The listing builds one solid part. Answer for the finished solid, in the listing's coordinates (mm). Round coordinates to 2 decimals unless told otherwise and drop trailing zeros. Write each loop counter-clockwise with the first axis right and the second up, starting at its lowest first coordinate (ties: lowest second). Pieces come first, ordered by that corner, then holes. Notation, with made-up numbers: M 68,-23.75 L 116,-23.75 A19 cw 116,-0.75 Z; hole C -16,46.25 d7. An arc over 180 degrees is marked long. One line per item, written item: value. Start each with the question number.
(1) Section D-D (z = -26.5) is taken. Determine the outline of the cut face in (x, y), plus the area to 3 significant figures.
(2) Section C-C (y = 14.25) is taken. Determine the outline of the cut face in (x, z).
(3) Section B-B (z = 0) is taken. Determine the outline of the cut face in (x, y).
(4) Consider probe 1 along Z at (x, y) = (0, 10.5); probe 2 along Z at (x, y) = (26, 16.25); probe 3 along X at (y, z) = (3.5, -16.5). Determine where each line is inside the solid, lowest interval first.
(5) Given P1, Ø3, axis at x = 0, z = -8, coming from the -Y side; P2, Ø8, axis at x = -32, y = 7, coming from the +Z side; P3, Ø2, axis at x = -11, y = 19.5, coming from the +Z side; P4, Ø3, axis at y = 16.5, z = -31.5, coming from the +X side, each flat-ended and moving along its own axis, determine where each tip first touches the part or whether it passes through.
(6) Section A-A (x = 0) is taken. Determine the outline of the cut face in (y, z).
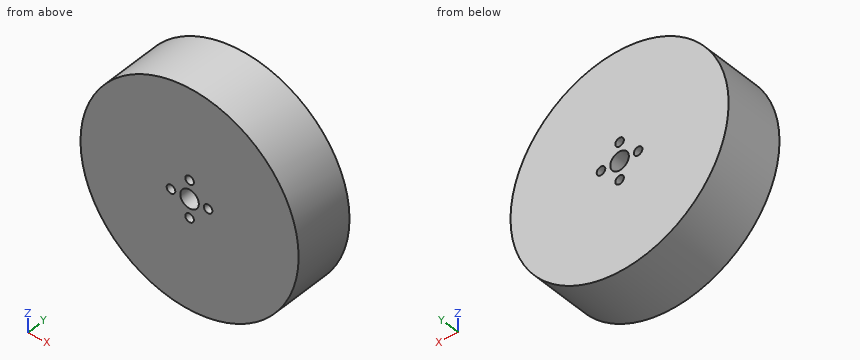
Autodesk Inventor part; units mm, degrees
ref_plane "YZ Plane" through (0, 0, 0) normal (1, 0, 0) x (0, 1, 0)
ref_plane "XZ Plane" through (0, 0, 0) normal (0, 1, 0) x (-1, 0, 0)
ref_plane "XY Plane" through (0, 0, 0) normal (0, 0, 1) x (1, 0, 0)
sketch "Sketch1" plane through (0, 0, 0) normal (0, 1, 0) x (-1, 0, 0)
  circle A0 centre (0, 0) radius 47
  circle A1 centre (0, 0) radius 4
  circle A2 centre (0, 8) radius 1.85
  circle A3 centre (-8, 0) radius 1.85
  circle A4 centre (8, 0) radius 1.85
  circle A5 centre (0, -8) radius 1.85
  dimension "d0" = 94
extrude "Extrusion2" add sketch "Sketch1" along normal blind 26
properties part number "AM Wheel"
Recorded:
1. outline: M -38.82,0 L 38.82,0 L 38.82,26 L -38.82,26 Z
1. area: 2,020 mm2
2. outline: C 0,0 d94; hole C -8,0 d3.7; hole C 0,0 d8; hole C 0,-8 d3.7; hole C 0,8 d3.7; hole C 8,0 d3.7
3. outline: M -47,0 L -9.85,0 L -9.85,26 L -47,26 Z; M -6.15,0 L -4,0 L -4,26 L -6.15,26 Z; M 4,0 L 6.15,0 L 6.15,26 L 4,26 Z; M 9.85,0 L 47,0 L 47,26 L 9.85,26 Z
4. probe 1: z = -47 to -9.85, -6.15 to -4, 4 to 6.15, 9.85 to 47
4. probe 2: z = -39.15 to 39.15
4. probe 3: x = -44.01 to 44.01
5. P1: passes through
5. P2: stops at z = 37.75
5. P3: stops at z = 45.92
5. P4: stops at x = 36.18
6. outline: M 0,-47 L 26,-47 L 26,-9.85 L 0,-9.85 Z; M 0,-6.15 L 26,-6.15 L 26,-4 L 0,-4 Z; M 0,4 L 26,4 L 26,6.15 L 0,6.15 Z; M 0,9.85 L 26,9.85 L 26,47 L 0,47 Z
